Autodesk Inventor part; units mm, degrees
ref_plane "YZ Plane" through (0, 0, 0) normal (1, 0, 0) x (0, 1, 0)
ref_plane "XZ Plane" through (0, 0, 0) normal (0, 1, 0) x (-1, 0, 0)
ref_plane "XY Plane" through (0, 0, 0) normal (0, 0, 1) x (1, 0, 0)
sketch "Sketch1" plane through (0, 0, 0) normal (0, 0, 1) x (1, 0, 0)
  line L0 (0, 0) -> (215.9, 0)
  line L1 (215.9, 0) -> (215.9, 152.4)
  line L2 (215.9, 152.4) -> (0, 152.4)
  line L3 (0, 152.4) -> (0, 0)
  dimension "d0" = 215.9
  dimension "d1" = 152.4
extrude "Extrusion1" add sketch "Sketch1" along normal blind 3.175
sketch "Sketch2" plane through (0, 0, 3.175) normal (0, 0, 1) x (1, 0, 0)
  line L0 (215.9, 152.4) -> (0, 152.4) construction
  line L1 (107.95, 152.4) -> (107.95, 0) construction
  line L2 (0, 0) -> (215.9, 0)
  point P0 (25.4, 59.8875)
  point P1 (76.2, 7.5)
  point P2 (190.5, 59.8875)
  point P3 (139.7, 7.5)
  dimension "d5" = 31.75
  dimension "d7" = 82.55
  dimension "d9" = 52.3875
  dimension "d10" = 7.5
hole "Hole1" at (25.4, 59.8875, 3.175) at (76.2, 7.5, 3.175) at (190.5, 59.8875, 3.175) at (139.7, 7.5, 3.175) direction (0, 0, -1) diameter 6.35 end through all
sketch "Sketch3" plane through (0, 0, 3.175) normal (0, 0, 1) x (1, 0, 0)
  line L0 (215.9, 152.4) -> (0, 152.4)
  line L1 (107.95, 152.4) -> (107.95, 0)
  line L2 (0, 0) -> (215.9, 0)
  circle A0 centre (25.4, 59.8875) radius 3.175
  circle A1 centre (76.2, 7.5) radius 3.175
  line L3 (25.4, 59.8875) -> (76.2, 7.5) construction
  line L4 (0.8957, 76.0359) -> (73.692, 0.9647)
  line L5 (0, 152.4) -> (0, 0)
  line L6 (0, 130.175) -> (0, 78.2462)
  line L7 (3.175, 133.35) -> (107.95, 133.35)
  line L8 (0, 133.35) -> (0, 125.3708)
  circle A2 centre (190.5, 59.8875) radius 3.175
  circle A3 centre (139.7, 7.5) radius 3.175
  line L9 (190.5, 59.8875) -> (139.7, 7.5) construction
  line L10 (215.0043, 76.0359) -> (142.208, 0.9647)
  line L11 (215.9, 152.4) -> (215.9, 78.2462)
  line L12 (215.9, 133.35) -> (215.9, 76.9596)
  line L13 (212.725, 133.35) -> (107.95, 133.35)
  line L14 (215.9, 130.175) -> (215.9, 125.3708)
  arc A4 (3.175, 133.35) -> (0, 130.175) centre (3.175, 130.175) ccw
  arc A5 (0, 78.2462) -> (0.8957, 76.0359) centre (3.175, 78.2462) ccw
  line L15 (75.9713, 0) -> (107.95, 0)
  line L16 (139.9287, 0) -> (107.95, 0)
  arc A6 (73.692, 0.9647) -> (75.9713, 0) centre (75.9713, 3.175) ccw
  arc A7 (139.9287, 0) -> (142.208, 0.9647) centre (139.9287, 3.175) ccw
  arc A8 (215.0043, 76.0359) -> (215.9, 78.2462) centre (212.725, 78.2462) ccw
  arc A9 (215.9, 130.175) -> (212.725, 133.35) centre (212.725, 130.175) ccw
  line L17 (215.9, 0) -> (215.9, 152.4)
  point P0 (74.6275, 0)
  point P1 (0, 76.9596)
  point P2 (77.9849, 0)
  dimension "d19" = 6.35
  dimension "d20" = 19.05
  dimension "d21" = 3.175
  dimension "d22" = 3.175
  dimension "d23" = 3.175
  dimension "d27" = 31.9787
  dimension "d28" = 31.9787
extrude "Extrusion2" cut sketch "Sketch3" against normal blind 3.175 contours L11 A9 L13 L1 L0 | L1 L7 A4 L5 L0 | L2 L5 A5 L4 A6 | A7 L10 A8 L12 L17 L2
sketch "Sketch4" plane through (0, 0, 3.175) normal (0, 0, 1) x (1, 0, 0)
  circle A0 centre (76.2059, 20.2) radius 3.175
  circle A1 centre (76.2, 7.5) radius 3.175
  line L0 (73.0309, 20.2015) -> (73.0254, 7.4505)
  circle A2 centre (76.2, 7.5) radius 3.175
  line L1 (79.3809, 20.2) -> (79.375, 7.4971)
  line L2 (3.175, 133.35) -> (212.725, 133.35)
  line L3 (107.95, 133.35) -> (107.95, 0) construction
  line L4 (75.9713, 0) -> (139.9287, 0)
  circle A3 centre (139.6941, 20.2) radius 3.175
  line L5 (142.8691, 20.2015) -> (142.8746, 7.4505)
  line L6 (136.5191, 20.2) -> (136.525, 7.5)
  circle A4 centre (76.2, 7.5) radius 3.175
  circle A5 centre (139.7, 7.5) radius 3.175
  circle A6 centre (139.7, 7.5) radius 3.175
  point P0 (0, 0)
  point P1 (136.525, 7.4971)
  dimension "d29" = 6.35
  dimension "d30" = 12.7
equation "\"d28\" = d27"
properties part number "new pulley plate"
Model file for the job. Use its own axes, mm. Give positions to 0.01 mm unless a question says otherwise; leave off trailing zeros. Loops run counter-clockwise (first coordinate to the right, second up) from the corner with the lowest first, then second, coordinate; pieces in that order, holes last. Notation, with made-up numbers: (65, 48.5) -> (90, 48.5) arc R13 ccw to (90, 63.5) -> close; hole circle Ø2 at (51.25, 59.25). An arc over 180 degrees is marked (long way). Use a Markdown table: item, result. Add a question column.
(1) Slice it at D-D on y = 24.5. List the corners of the cut face in (x, z) (3 decimals), and give its area (3 significant figures).
(2) Slice it at A-A on z = 0.85. Give the number of separate pieces and of enclosed holes in the cut face, and give its area (3 significant figures).
(3) Slice it at B-B on y = 7.5. List the corners of the cut face in (x, z) (3 decimals), and give its area (3 significant figures).
(4) Mould opens along Y. For faces 1 (the cylindrical face through (189.55, 56.86, 1.57)), 2 (the flat face through (106, 82, 0)), 3 (the flat face through (179.12, 39.03, 1.61)), 4 (the cylindrical face through (136.55, 7.91, 1.57)) say: +Y half, -Y half, draft (parallel to the pull), parting line (faces both ways), or undercut.
(5) Wall check: line 1 along X through (y, z) = (9, 1.35); line 2 along X through (y, z) = (7.5, 1.05) (3 decimals); line 3 along Y through (x, z) = (139.7, 1.2) (3 decimals). Give the ranges that are in metal, low to high.
Filled sheet:
| question | item | result |
|---|---|---|
| 1 | outline | (50.87, 0) -> (165.03, 0) -> (165.03, 3.175) -> (50.87, 3.175) -> close |
| 1 | area | 362 mm2 |
| 2 | separate pieces | 1 |
| 2 | enclosed holes | 4 |
| 2 | area | 22,900 mm2 |
| 3 | outline | (67.355, 0) -> (73.025, 0) -> (73.025, 3.175) -> (67.355, 3.175) -> close; (79.375, 0) -> (136.525, 0) -> (136.525, 3.175) -> (79.375, 3.175) -> close; (142.875, 0) -> (148.545, 0) -> (148.545, 3.175) -> (142.875, 3.175) -> close |
| 3 | area | 217 mm2 |
| 4 | face 1 | undercut |
| 4 | face 2 | draft |
| 4 | face 3 | -Y half |
| 4 | face 4 | undercut |
| 5 | line 1 | 65.9 to 73.4, 79 to 136.9, 142.5 to 150 |
| 5 | line 2 | 67.355 to 73.025, 79.375 to 136.525, 142.875 to 148.545 |
| 5 | line 3 | 0 to 4.325, 10.675 to 133.35 |
